Source: CAD feature listing. Evaluate the final solid. Frame: model axes, mm. Round coordinates to 2 decimals unless told otherwise and drop trailing zeros. Loops run counter-clockwise (first coordinate to the right, second up) from the corner with the lowest first, then second, coordinate; pieces in that order, holes last.
(1) Section C-C, the plane y = 444.5. Return the cut outline in (x, z), plus the area to 3 significant figures.
(2) Mould query, pull axis X, two halves, no side actions, for faces 1 (the flat face through (150, 736.6, -155)), 2 (the cylindrical face through (168.919, 370.112, -154.534)), 3 (the flat face through (0, 389, -150)). Classes: pulls with the +X half, pulls with the -X half, needs draft (parallel to the pull), parting line crosses it, or undercut.
(3) Section A-A, the plane x = 152.4. Return the cut outline in (y, z), plus the area to 3 significant figures.
(4) Section B-B, the plane z = -53. Return the cut outline in (x, y), plus the area to 3 significant figures.
(5) Section D-D, the plane x = 265. Return the cut outline in (y, z).
(6) Material intervals for probe 1 along Y at (x, z) = (152.4, -99); probe 2 along X at (y, z) = (414, -97); probe 3 along X at (y, z) = (444, -233), sorted ascending.
(7) First-contact query: pin 1 Ø1.5 at (x, z) = (31, -179.5) entering from -Y. Flat tip, straight axial feed; report the tip coordinate or a pass-through.
```python
from build123d import *

# Parameters (mm, degrees)
SKETCH1_W           = 304.8
SKETCH1_H           = 304.8
BOSS_EXTRUDE1_DEPTH = 736.6
CUT_EXTRUDE1_REACH  = 855.455
SKETCH2_R           = 76.2
FILLET1_R           = 50.8


with BuildPart() as part:
    # Sketch1 → Boss-Extrude1 (new body)
    with BuildSketch(Plane(origin=(0, 0, 0), x_dir=(1, 0, 0), z_dir=(0, 1, 0))):
        with Locations((152.4, 152.4)):
            Rectangle(SKETCH1_W, SKETCH1_H)
    extrude(amount=BOSS_EXTRUDE1_DEPTH)

    # Sketch2 → Cut-Extrude1 (cut, up to next)
    with BuildSketch(Plane(origin=(0, 0, -304.8), x_dir=(-1, 0, 0), z_dir=(0, 0, -1)), mode=Mode.PRIVATE) as cut_extrude1_sk1:
        with Locations((-152.4, 444.5)):
            Circle(SKETCH2_R)
    cut_extrude1_tool1 = extrude(cut_extrude1_sk1.sketch, amount=-CUT_EXTRUDE1_REACH, mode=Mode.PRIVATE) & part.part
    # Sketch2 → Cut-Extrude1 (cut, up to next)
    with BuildSketch(Plane(origin=(0, 0, -304.8), x_dir=(-1, 0, 0), z_dir=(0, 0, -1)), mode=Mode.PRIVATE) as cut_extrude1_sk2:
        Polygon((-304.8, 736.6), (-231.279579983, 0), (-304.8, 0), align=None)
    cut_extrude1_tool2 = extrude(cut_extrude1_sk2.sketch, amount=-CUT_EXTRUDE1_REACH, mode=Mode.PRIVATE) & part.part
    add(cut_extrude1_tool1.solids().sort_by_distance((152.4, 444.5, -304.8))[0], mode=Mode.SUBTRACT)
    add(cut_extrude1_tool2.solids().sort_by_distance((280.293193, 245.533333, -304.8))[0], mode=Mode.SUBTRACT)

    # Fillet1
    fillet1_edges = [part.edges().sort_by_distance(p)[0] for p in [
        (231.279579983, 0, -152.4),
        (0, 0, -152.4),
    ]]
    fillet(fillet1_edges, radius=FILLET1_R)


solid = part.part
```
Output values:
1. outline: (0, -304.8) - (76.2, -304.8) - (76.2, 0) - (0, 0) - close; (228.6, -304.8) - (275.65, -304.8) - (275.65, 0) - (228.6, 0) - close
1. area: 37,600 mm2
2. face 1: needs draft
2. face 2: undercut
2. face 3: pulls with the -X half
3. outline: (0, -304.8) - (368.3, -304.8) - (368.3, 0) - (0, 0) - close; (520.7, -304.8) - (736.6, -304.8) - (736.6, 0) - (520.7, 0) - close
3. area: 178,000 mm2
4. outline: (0, 50.8) arc R50.8 ccw to (50.8, 0) - (185.3, 0) arc R50.8 ccw to (235.85, 45.75) - (304.8, 736.6) - (0, 736.6) - close; hole circle Ø152.4 at (152.4, 444.5)
4. area: 178,000 mm2
5. outline: (337.84, -304.8) - (736.6, -304.8) - (736.6, 0) - (337.84, 0) - close
6. probe 1: y = 0 to 368.3, 520.7 to 736.6
6. probe 2: x = 0 to 82.57, 222.23 to 272.6
6. probe 3: x = 0 to 76.2, 228.6 to 275.6
7. pin 1: stops at y = 3.71
